```python
from build123d import *

# Parameters (mm, degrees)
SKETCH1_R           = 25
SKETCH1_R_2         = 12.5
BOSS_EXTRUDE2_DEPTH = 3
BOSS_EXTRUDE3_DEPTH = 1
CIRPATTERN1_COUNT   = 24


with BuildPart() as part:
    # Sketch1 → Boss-Extrude2 (new, symmetric)
    with BuildSketch(Plane(origin=(0, 0, 0), x_dir=(1, 0, 0), z_dir=(0, 1, 0))):
        with Locations(Location((0, 0, 0), (0, 0, 270))):
            Circle(SKETCH1_R)
        with Locations(Location((0, 0, 0), (0, 0, 270))):
            Circle(SKETCH1_R_2, mode=Mode.SUBTRACT)
    extrude(amount=BOSS_EXTRUDE2_DEPTH, both=True)

    # Sketch4 → Boss-Extrude3 (add, symmetric)
    with BuildSketch(Plane(origin=(0, 0, 0), x_dir=(1, 0, 0), z_dir=(0, 1, 0))):
        Polygon((0, 30), (-3.612358793, 24.73764063), (0, 25), (3.394844565, 24.768428097), align=None)
    boss_extrude3 = extrude(amount=BOSS_EXTRUDE3_DEPTH, both=True)

    # CirPattern1: Boss-Extrude3 ×24 about axis
    cirpattern1_axis = Axis((0, 0, 0), (0, 1, 0))
    for i in range(1, CIRPATTERN1_COUNT):
        add(boss_extrude3.rotate(cirpattern1_axis, i * 360 / CIRPATTERN1_COUNT))


solid = part.part
```
Here's how the part is built. I have some questions about the finished solid (model axes, mm). A direction names the side the tool comes from. Give positions to 0.01 mm unless a question says otherwise; leave off trailing zeros. Loops run counter-clockwise (first coordinate to the right, second up) from the corner with the lowest first, then second, coordinate; pieces in that order, holes last. Notation, with made-up numbers: (6.5, 85) -> (41.5, 85) arc R23 ccw to (41.5, 110) -> close; hole circle Ø7 at (15, 87.5). An arc over 180 degrees is marked (long way). Use one line per item in the form item = value. Start each with the question number.
1) Which directions (+Z, -Z, +X, -X, +Y, -Y) give clear straight access to the entire face, cutting with the end or side of a thin tool? Please do faces 1 (the face through (-20.593, 0.014, 18.3)), 2 (the face through (-5.51, 0.01, 27.05)), 3 (the face through (-5.55, 0.01, -26.98)).
2) For P1, Ø3, axis at x = 4.5, y = -2, coming from the +Z side; P2, Ø3, axis at y = -0.5, z = -5, coming from the +X side; P3, Ø1.5, axis at y = 1, z = 12, coming from the +X side, each with a flat end and sliding along its axis, tell me the tip position at first contact or that it passes through.
3) Imagine slicing it at B-B (x = -5.5). Please give me the cut outline in (y, z).
4) Imagine slicing it at A-A (z = 5). Please give me the cut outline in (x, y).
5) Imagine slicing it at C-C (y = 1.8). Please give me the cut outline in (x, z), then the cut area to 3 significant figures.
6) Thinking about a two-plate mould opening in X: for faces 4 (the face through (18.3, 0.01, -20.67)), 5 (the face through (-18.3, 0.014, -20.593)), 6 (the face through (23.007, 0.014, 15.155)), 7 (the face through (-27.558, 0.014, 1.677)), which applies, +X half, -X half, draft (parallel to the pull), parting line (faces both ways), or undercut?
7) Imagine slicing it at D-D (x = 14). Please give me the cut outline in (y, z).
8) Please list where these lines run through material, in increasing order: line 1 along Z through (x, y) = (23.5, -0.8); line 2 along X through (y, z) = (-2, 20); line 3 along X through (y, z) = (0.4, -6).
Check values:
q1.face_1 = -X, +Y, -Y
q1.face_2 = +Z, +Y, -Y
q1.face_3 = -Z, +Y, -Y
q2.P1 = 27.04
q2.P2 = 27.84
q2.P3 = 24.91
q3.outline = (-3, -24.39) -> (-1, -24.39) -> (-1, -26.94) -> (1, -26.94) -> (1, -24.39) -> (3, -24.39) -> (3, -11.22) -> (-3, -11.22) -> close; (-3, 11.22) -> (3, 11.22) -> (3, 24.39) -> (1, 24.39) -> (1, 27.04) -> (-1, 27.04) -> (-1, 24.39) -> (-3, 24.39) -> close
q4.outline = (-26.49, -1) -> (-24.49, -1) -> (-24.49, -3) -> (-11.46, -3) -> (-11.46, 3) -> (-24.49, 3) -> (-24.49, 1) -> (-26.49, 1) -> close; (11.46, -3) -> (24.49, -3) -> (24.49, -1) -> (26.61, -1) -> (26.61, 1) -> (24.49, 1) -> (24.49, 3) -> (11.46, 3) -> close
q5.outline = circle Ø50 at (0, 0); hole circle Ø25 at (0, 0)
q5.area = 1,470 mm^2
q6.face_4 = undercut
q6.face_5 = undercut
q6.face_6 = +X half
q6.face_7 = -X half
q7.outline = (-3, -20.71) -> (-1, -20.71) -> (-1, -25.5) -> (1, -25.5) -> (1, -20.71) -> (3, -20.71) -> (3, 20.71) -> (1, 20.71) -> (1, 25.47) -> (-1, 25.47) -> (-1, 20.71) -> (-3, 20.71) -> close
q8.line_1 = -15.19 to -10.14, -9.7 to 9.54, 9.81 to 15.13
q8.line_2 = -15 to 15
q8.line_3 = -27.47 to -10.97, 10.97 to 27.39
